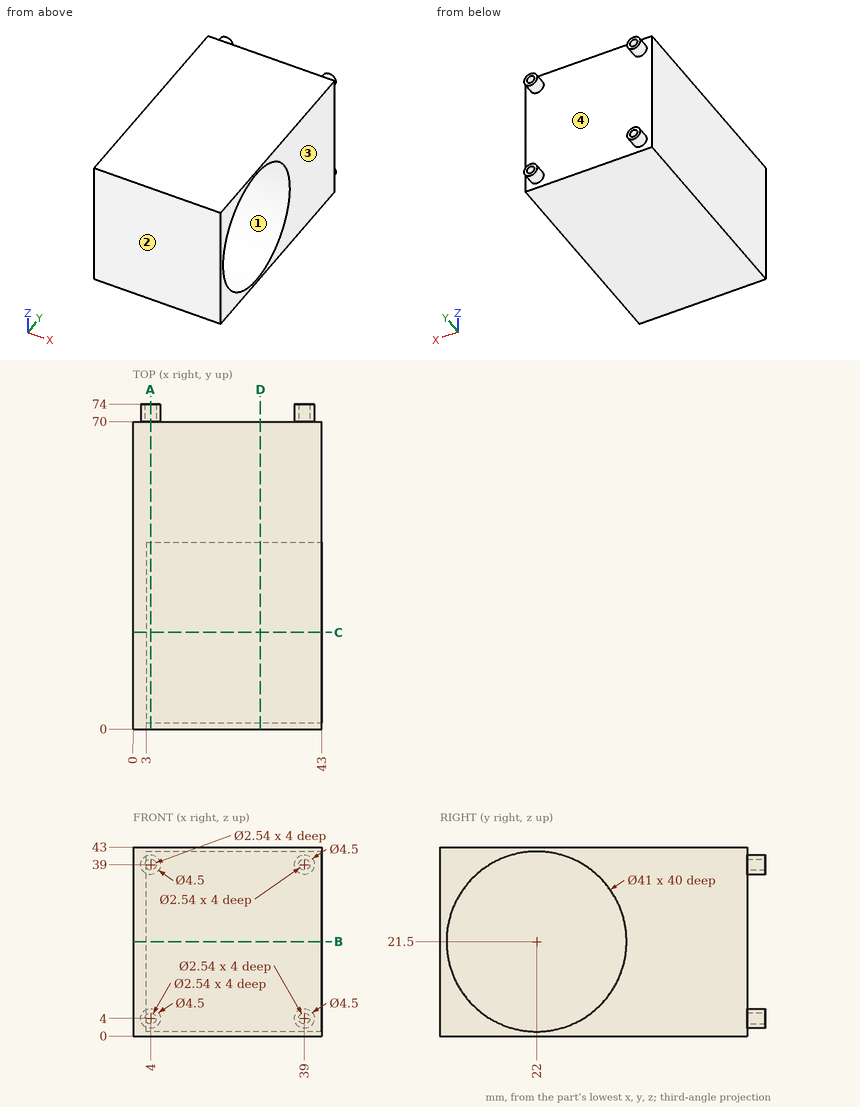
Here's the drawing with two shaded views (mm, measured from the low corner). I have some questions. Coordinates: 2 decimals unless noted, no trailing zeros. Order: outer loops, then holes, each group sorted by start corner. A loop starts at its lowest first (then second) coordinate and runs counter-clockwise, first axis right, second up.
Item 1: I need wall thicknesses on probe 1 along X at (y, z) = (72.8, 4); probe 2 along Y at (x, z) = (28, 28.5); probe 3 along Z at (x, y) = (10, 21.5). Which ranges of each line are inside material? Lowest first, please.
Response values:
probe 1: x = 1.75 to 2.73, 5.27 to 6.25, 36.75 to 37.73, 40.27 to 41.25
probe 2: y = 0 to 2.73, 41.27 to 70
probe 3: z = 0 to 1.01, 41.99 to 43
Item 2: If we section it at D-D, the plane x = 29: List the corners of the cut face in (y, z) for me, then the cut area to 3 significant figures.
Response values:
outline: (0, 0) - (70, 0) - (70, 43) - (0, 43) - close; hole circle Ø41 at (22, 21.5)
area: 1,690 mm2
Item 3: If we section it at A-A, the plane x = 4: List the corners of the cut face in (y, z) for me, then the cut area to 3 significant figures.
Response values:
outline: (0, 0) - (70, 0) - (70, 1.75) - (74, 1.75) - (74, 2.73) - (70, 2.73) - (70, 5.27) - (74, 5.27) - (74, 6.25) - (70, 6.25) - (70, 36.75) - (74, 36.75) - (74, 37.73) - (70, 37.73) - (70, 40.27) - (74, 40.27) - (74, 41.25) - (70, 41.25) - (70, 43) - (0, 43) - close; hole circle Ø41 at (22, 21.5)
area: 1,710 mm2
Item 4: Thinking about a two-plate mould opening in Y: for the marked faces 1, 2, 3 and 4, which applies, pulls with the +Y half, pulls with the -Y half, needs draft (parallel to the pull), parting line crosses it, or undercut?
Response values:
face 1: undercut
face 2: pulls with the -Y half
face 3: needs draft
face 4: pulls with the +Y half
Item 5: If we section it at C-C, the plane y = 22: List the corners of the cut face in (x, z) for me.
Response values:
outline: (0, 0) - (43, 0) - (43, 1) - (3, 1) - (3, 42) - (43, 42) - (43, 43) - (0, 43) - close
Item 6: If we section it at B-B, the plane z = 21.5: List the corners of the cut face in (x, y) for me, then the cut area to 3 significant figures.
Response values:
outline: (0, 0) - (43, 0) - (43, 1.5) - (3, 1.5) - (3, 42.5) - (43, 42.5) - (43, 70) - (0, 70) - close
area: 1,370 mm2
Item 7: I'm going to push flat-ended pins straight in: pin 1 Ø20.5 at (y, z) = (18, 17.5) entering from +X; pin 2 Ø1.3 at (x, z) = (39, 39.5) entering from +Y. Where does each tip first touch, or does it pass through?
Response values:
pin 1: stops at x = 3
pin 2: stops at y = 70
